```python
from build123d import *

# Parameters (mm, degrees)
EXTRUDE_1_DEPTH      = 1
EXTRUDE_1_DEPTH_BACK = 1
SKETCH_2_R           = 4.25
SKETCH_2_R_2         = 3.25
EXTRUDE_2_DEPTH      = 9
SKETCH_3_R           = 1.1
CUT_EXTRUDE_1_DEPTH  = 14.948989624
SKETCH_8_R           = 2
CUT_EXTRUDE_3_DEPTH  = 1
SKETCH_4_R           = 4
EXTRUDE_1_2_DEPTH    = 6.5
SKETCH_5_OUTSIDE_W   = 26.596
SKETCH_5_OUTSIDE_H   = 17.016
SKETCH_5_OUTSIDE_R   = 3.9
CUT_EXTRUDE_2_DEPTH  = 8


with BuildPart() as part:
    # 草图1 → Extrude 1 (new, two sides: drawn at the far end of the back side and taken through both)
    with BuildSketch(Plane(origin=(0, 0, 0), x_dir=(1, 0, 0), z_dir=(0, 1, 0)).offset(-EXTRUDE_1_DEPTH_BACK)):
        with BuildLine():
            Line((-7.5, 4.75), (7.5, 4.75))
            ThreePointArc((7.5, 4.75), (9.540011086, 0), (7.5, -4.75))
            Line((7.5, -4.75), (-7.5, -4.75))
            ThreePointArc((-7.5, -4.75), (-9.540011086, 0), (-7.5, 4.75))
        make_face()
    extrude(amount=EXTRUDE_1_DEPTH + EXTRUDE_1_DEPTH_BACK)

    # 草图2 → Extrude 2 (add)
    with BuildSketch(Plane(origin=(0, 1, 0), x_dir=(-1, 0, 0), z_dir=(0, 1, 0))):
        with Locations(Location((0, 0, 0), (0, 0, 270))):
            Circle(SKETCH_2_R)
        with Locations(Location((0, 0, 0), (0, 0, 90))):
            Circle(SKETCH_2_R_2, mode=Mode.SUBTRACT)
    extrude(amount=EXTRUDE_2_DEPTH)

    # 草图3 → 切除-拉伸1 (cut, through all)
    with BuildSketch(Plane(origin=(0, 1, 0), x_dir=(-1, 0, 0), z_dir=(0, 1, 0))):
        with Locations(Location((-6.75, 0, 0), (0, 0, 90))):
            Circle(SKETCH_3_R)
        with Locations(Location((6.75, 0, 0), (0, 0, 270))):
            Circle(SKETCH_3_R)
    extrude(amount=-CUT_EXTRUDE_1_DEPTH, mode=Mode.SUBTRACT)

    # 草图8 → 切除-拉伸3 (cut)
    with BuildSketch(Plane(origin=(0, 1, 0), x_dir=(1, 0, 0), z_dir=(0, 1, 0))):
        with Locations(Location((-6.75, 0, 0), (0, 0, 270))):
            Circle(SKETCH_8_R)
        with Locations(Location((6.75, 0, 0), (0, 0, 270))):
            Circle(SKETCH_8_R)
    extrude(amount=-CUT_EXTRUDE_3_DEPTH, mode=Mode.SUBTRACT)

    # 草图4 → Extrude 1 2 (add)
    with BuildSketch(Plane.XZ.offset(1)):
        with Locations(Location((0, 0, 0), (0, 0, 90))):
            Circle(SKETCH_4_R)
    extrude(amount=EXTRUDE_1_2_DEPTH)

    # 草图5 outside → 切除-拉伸2 (cut)
    with BuildSketch(Plane(origin=(0, 10, 0), x_dir=(1, 0, 0), z_dir=(0, 1, 0))):
        Rectangle(SKETCH_5_OUTSIDE_W, SKETCH_5_OUTSIDE_H)
        with Locations(Location((0, 0, 0), (0, 0, 270))):
            Circle(SKETCH_5_OUTSIDE_R, mode=Mode.SUBTRACT)
    extrude(amount=-CUT_EXTRUDE_2_DEPTH, mode=Mode.SUBTRACT)


solid = part.part
```
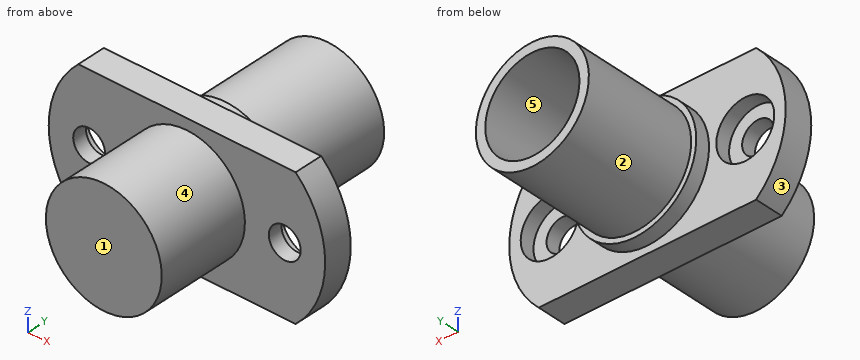
Read the model definition and answer for the solid it produces. Units are mm, in the model's axes. Face numbers are marked on the shaded views. A direction names the side the tool comes from. Round coordinates to 2 decimals unless told otherwise and drop trailing zeros. Write each loop counter-clockwise with the first axis right and the second up, starting at its lowest first coordinate (ties: lowest second). Pieces come first, ordered by that corner, then holes. Notation, with made-up numbers: (63.25, -33) - (104.25, -33) arc R18 ccw to (104.25, 2) - close; hole circle Ø5 at (-16.5, 39). An arc over 180 degrees is marked (long way). One line per item, written item: value.
Q1. Straight lines are drawn through the part: line 1 (X direction, y = 0.65, z = 0); line 2 (X direction, y = -0.25, z = 0); line 3 (Z direction, x = -6.75, y = -0.55). For each, find the intervals that lie inside material, in ascending order. Write a range as from..to.
The answers:
line 1: x = -9.54..-8.75, -4.75..4.75, 8.75..9.54
line 2: x = -9.54..-7.85, -5.65..5.65, 7.85..9.54
line 3: z = -4.75..-1.1, 1.1..4.75
Q2. Find section B-B (z = -2.5). Determine the outline of the cut face in (x, y), and give its area (3 significant figures).
The answers:
outline: (-9.04, -1) - (-3.12, -1) - (-3.12, -7.5) - (3.12, -7.5) - (3.12, -1) - (9.04, -1) - (9.04, 1) - (3.44, 1) - (3.44, 2) - (2.99, 2) - (2.99, 10) - (2.08, 10) - (2.08, 1) - (-2.08, 1) - (-2.08, 10) - (-2.99, 10) - (-2.99, 2) - (-3.44, 2) - (-3.44, 1) - (-9.04, 1) - close
area: 94.2 mm2
Q3. Which of the six approach directions +Z, -Z, +X, -X, +Y, -Y give full straight-line access (tool end or side, diameter ignored) to the marked faces 1 and 2?
The answers:
face 1: +Z, -Z, +X, -X, -Y
face 2: +Y
Q4. Find section A-A (x = 6.75). Determine the outline of the cut face in (y, z), and give its area (3 significant figures).
The answers:
outline: (-1, -4.75) - (1, -4.75) - (1, -2) - (0, -2) - (0, -1.1) - (-1, -1.1) - close; (-1, 1.1) - (0, 1.1) - (0, 2) - (1, 2) - (1, 4.75) - (-1, 4.75) - close
area: 12.8 mm2
Q5. Find section C-C (x = 0). Determine the outline of the cut face in (y, z), and give its area (3 significant figures).
The answers:
outline: (-7.5, -4) - (-1, -4) - (-1, -4.75) - (1, -4.75) - (1, -4.25) - (2, -4.25) - (2, -3.9) - (10, -3.9) - (10, -3.25) - (1, -3.25) - (1, 3.25) - (10, 3.25) - (10, 3.9) - (2, 3.9) - (2, 4.25) - (1, 4.25) - (1, 4.75) - (-1, 4.75) - (-1, 4) - (-7.5, 4) - close
area: 83.4 mm2
Q6. Find section D-D (y = -3.5). Determine the outline of the cut face in (x, z), and give its area (3 significant figures).
The answers:
outline: circle Ø8 at (0, 0)
area: 50.3 mm2
Q7. For a pull along X with two mould halves and no side action, classify the marked faces 3, 4 and 5 as pulls with the +X half, pulls with the -X half, needs draft (parallel to the pull), parting line crosses it, or undercut.
The answers:
face 3: pulls with the -X half
face 4: parting line crosses it
face 5: undercut
Q8. Each of these flat-tipped pins is pushed along its axis until it touches: P1, Ø3, axis at y = 2, z = -1.5, coming from the -X side; P2, Ø1, axis at x = 1.5, y = 4.5, coming from the +Z side; P3, Ø3.5, axis at x = -6.75, z = 0, coming from the -Y side; P4, Ø2, axis at x = 6.75, z = 0, coming from the -Y side. Where does it stop, or does it pass through?
The answers:
P1: stops at x = -9.53
P2: stops at z = 3.77
P3: stops at y = -1
P4: passes through
